Verification items for the finished model (mm, model axes). Face numbers are marked on the shaded views. A direction names the side the tool comes from. Round coordinates to 2 decimals unless told otherwise and drop trailing zeros. Write each loop counter-clockwise with the first axis right and the second up, starting at its lowest first coordinate (ties: lowest second). Pieces come first, ordered by that corner, then holes. Notation, with made-up numbers: M -18.5,49 L 21.5,49 A32 cw 21.5,77 Z; hole C 83.5,-21.75 d10. An arc over 180 degrees is marked long. One line per question, with ' | ' between items.
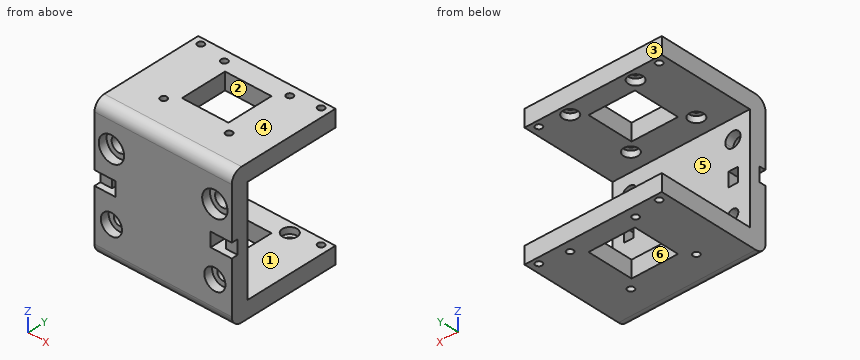
from build123d import *

# Parameters (mm, degrees)
F0_W      = 65
F0_H      = 50
F0_W_2    = 45
F0_H_2    = 6.7
F1_DEPTH  = 8
F2_R      = 6
F2_R_2    = 3.6
F2_R_3    = 5
F2_R_4    = 2.55
F3_DEPTH  = 4
F4_W      = 5.5
F4_H      = 6.7
F5_DEPTH  = 3
F6_DEPTH  = 8
F7_DEPTH  = 8
F8_W      = 65
F8_H      = 8
F9_DEPTH  = 45
F10_W     = 22
F10_H     = 22
F10_R     = 1.55
F11_DEPTH = 100
F12_R     = 3.5
F12_R_2   = 1.55
F13_DEPTH = 3
F14_R     = 3.5
F14_R_2   = 1.55
F15_DEPTH = 3
F16_R     = 5


with BuildPart() as f1:
    # F0 (on Front) → F1 (new body)
    with BuildSketch(Plane.XZ):
        Rectangle(F0_W, F0_H)
        with BuildLine():
            ThreePointArc((-24.5, 12.35), (-27.0455844123, 18.4955844123), (-20.9, 15.95))
            Line((-20.9, 15.95), (20.9, 15.95))
            ThreePointArc((20.9, 15.95), (24.5, 19.55), (28.1, 15.95))
            ThreePointArc((28.1, 15.95), (27.0455844123, 13.4044155877), (24.5, 12.35))
            Line((24.5, 12.35), (24.5, 3.35))
            Line((24.5, 3.35), (27, 3.35))
            Line((27, 3.35), (27, -3.35))
            Line((27, -3.35), (24.5, -3.35))
            Line((24.5, -3.35), (24.5, -13.4))
            ThreePointArc((24.5, -13.4), (26.303122292, -14.146877708), (27.05, -15.95))
            ThreePointArc((27.05, -15.95), (24.5, -18.5), (21.95, -15.95))
            Line((21.95, -15.95), (-21.95, -15.95))
            ThreePointArc((-21.95, -15.95), (-26.303122292, -17.753122292), (-24.5, -13.4))
            Line((-24.5, -13.4), (-24.5, -3.35))
            Line((-24.5, -3.35), (-27, -3.35))
            Line((-27, -3.35), (-27, 3.35))
            Line((-27, 3.35), (-24.5, 3.35))
            Line((-24.5, 3.35), (-24.5, 12.35))
        make_face(mode=Mode.SUBTRACT)
        with BuildLine():
            Line((20.9, 15.95), (-20.9, 15.95))
            ThreePointArc((-20.9, 15.95), (-21.9544155877, 13.4044155877), (-24.5, 12.35))
            Line((-24.5, 12.35), (-24.5, 3.35))
            Line((-24.5, 3.35), (-22.5, 3.35))
            Line((-22.5, 3.35), (22.5, 3.35))
            Line((22.5, 3.35), (24.5, 3.35))
            Line((24.5, 3.35), (24.5, 12.35))
            ThreePointArc((24.5, 12.35), (21.9544155877, 13.4044155877), (20.9, 15.95))
        make_face()
        with BuildLine():
            Line((-22.5, -3.35), (-24.5, -3.35))
            Line((-24.5, -3.35), (-24.5, -13.4))
            ThreePointArc((-24.5, -13.4), (-22.696877708, -14.146877708), (-21.95, -15.95))
            Line((-21.95, -15.95), (21.95, -15.95))
            ThreePointArc((21.95, -15.95), (22.696877708, -14.146877708), (24.5, -13.4))
            Line((24.5, -13.4), (24.5, -3.35))
            Line((24.5, -3.35), (22.5, -3.35))
            Line((22.5, -3.35), (-22.5, -3.35))
        make_face()
        Rectangle(F0_W_2, F0_H_2)
    extrude(amount=F1_DEPTH)

    # F2 (on face) → F3 (cut)
    with BuildSketch(Plane.XZ.offset(8)):
        with Locations((24.5, 15.95)):
            Circle(F2_R)
        with Locations((24.5, 15.95)):
            Circle(F2_R_2, mode=Mode.SUBTRACT)
        with Locations((-24.5, 15.95)):
            Circle(F2_R)
        with Locations((-24.5, 15.95)):
            Circle(F2_R_2, mode=Mode.SUBTRACT)
        with Locations((-24.5, -15.95)):
            Circle(F2_R_3)
        with Locations((-24.5, -15.95)):
            Circle(F2_R_4, mode=Mode.SUBTRACT)
        with Locations((24.5, -15.95)):
            Circle(F2_R_3)
        with Locations((24.5, -15.95)):
            Circle(F2_R_4, mode=Mode.SUBTRACT)
    extrude(amount=-F3_DEPTH, mode=Mode.SUBTRACT)

    # F4 (on face) → F5 (cut)
    with BuildSketch(Plane.XZ.offset(8)):
        with Locations((29.75, 0)):
            Rectangle(F4_W, F4_H)
        with Locations((-29.75, 0)):
            Rectangle(F4_W, F4_H)
    extrude(amount=-F5_DEPTH, mode=Mode.SUBTRACT)

    # F6 (add): a face of the model
    f6_faces = [f1.faces().sort_by_distance(p)[0] for p in [
        (0, -4, -25),
    ]]
    extrude(f6_faces, amount=F6_DEPTH)

    # F7 (add): a face of the model
    f7_faces = [f1.faces().sort_by_distance(p)[0] for p in [
        (0, -4, 25),
    ]]
    extrude(f7_faces, amount=F7_DEPTH)

    # F8 (on face) → F9 (join)
    with BuildSketch(Plane(origin=(0, 0, 0), x_dir=(-1, 0, 0), z_dir=(0, 1, 0))):
        with Locations((0, 29)):
            Rectangle(F8_W, F8_H)
        with Locations((0, -29)):
            Rectangle(F8_W, F8_H)
    extrude(amount=F9_DEPTH)

    # F10 (on face) → F11 (cut)
    with BuildSketch(Plane.XY.offset(33)):
        with BuildLine():
            Line((15.5, 9), (13.95, 9))
            ThreePointArc((13.95, 9), (15.5, 7.45), (17.05, 9))
            ThreePointArc((17.05, 9), (16.5960155108, 10.0960155108), (15.5, 10.55))
            Line((15.5, 10.55), (15.5, 9))
        make_face()
        with BuildLine():
            ThreePointArc((15.5, 10.55), (14.4039844892, 10.0960155108), (13.95, 9))
            Line((13.95, 9), (15.5, 9))
            Line((15.5, 9), (15.5, 10.55))
        make_face()
        with BuildLine():
            ThreePointArc((-15.5, 10.55), (-16.5960155108, 7.9039844892), (-13.95, 9))
            Line((-13.95, 9), (-15.5, 9))
            Line((-15.5, 9), (-15.5, 10.55))
        make_face()
        with BuildLine():
            Line((-15.5, 9), (-13.95, 9))
            ThreePointArc((-13.95, 9), (-14.4039844892, 10.0960155108), (-15.5, 10.55))
            Line((-15.5, 10.55), (-15.5, 9))
        make_face()
        with BuildLine():
            Line((15.5, 40), (15.5, 38.45))
            ThreePointArc((15.5, 38.45), (16.5960155108, 38.9039844892), (17.05, 40))
            ThreePointArc((17.05, 40), (15.5, 41.55), (13.95, 40))
            Line((13.95, 40), (15.5, 40))
        make_face()
        with BuildLine():
            ThreePointArc((13.95, 40), (14.4039844892, 38.9039844892), (15.5, 38.45))
            Line((15.5, 38.45), (15.5, 40))
            Line((15.5, 40), (13.95, 40))
        make_face()
        with BuildLine():
            ThreePointArc((-13.95, 40), (-16.5960155108, 41.0960155108), (-15.5, 38.45))
            Line((-15.5, 38.45), (-15.5, 40))
            Line((-15.5, 40), (-13.95, 40))
        make_face()
        with BuildLine():
            Line((-15.5, 40), (-15.5, 38.45))
            ThreePointArc((-15.5, 38.45), (-14.4039844892, 38.9039844892), (-13.95, 40))
            Line((-13.95, 40), (-15.5, 40))
        make_face()
        with Locations((0, 24.5)):
            Rectangle(F10_W, F10_H)
        with Locations((28.5, 42)):
            Circle(F10_R)
        with BuildLine():
            ThreePointArc((-26.95, 42), (-28.5, 43.55), (-30.05, 42))
            ThreePointArc((-30.05, 42), (-28.5, 40.45), (-26.95, 42))
        make_face()
    extrude(amount=-F11_DEPTH, mode=Mode.SUBTRACT)

    # F12 (on face) → F13 (cut)
    with BuildSketch(Plane(origin=(0, 0, 25), x_dir=(1, 0, 0), z_dir=(0, 0, -1))):
        with Locations((-15.5, -40)):
            Circle(F12_R)
        with Locations((-15.5, -40)):
            Circle(F12_R_2, mode=Mode.SUBTRACT)
        with Locations((-15.5, -9)):
            Circle(F12_R)
        with Locations((-15.5, -9)):
            Circle(F12_R_2, mode=Mode.SUBTRACT)
        with Locations((15.5, -9)):
            Circle(F12_R)
        with Locations((15.5, -9)):
            Circle(F12_R_2, mode=Mode.SUBTRACT)
        with Locations((15.5, -40)):
            Circle(F12_R)
        with Locations((15.5, -40)):
            Circle(F12_R_2, mode=Mode.SUBTRACT)
    extrude(amount=-F13_DEPTH, mode=Mode.SUBTRACT)

    # F14 (on face) → F15 (cut)
    with BuildSketch(Plane.XY.offset(-25)):
        with Locations((15.5, 9)):
            Circle(F14_R)
        with Locations((15.5, 9)):
            Circle(F14_R_2, mode=Mode.SUBTRACT)
        with Locations((15.5, 40)):
            Circle(F14_R)
        with Locations((15.5, 40)):
            Circle(F14_R_2, mode=Mode.SUBTRACT)
        with Locations((-15.5, 40)):
            Circle(F14_R)
        with Locations((-15.5, 40)):
            Circle(F14_R_2, mode=Mode.SUBTRACT)
        with Locations((-15.5, 9)):
            Circle(F14_R)
        with Locations((-15.5, 9)):
            Circle(F14_R_2, mode=Mode.SUBTRACT)
    extrude(amount=-F15_DEPTH, mode=Mode.SUBTRACT)

    # F16
    f16_edges = [f1.edges().sort_by_distance(p)[0] for p in [
        (0, -8, -33),
        (0, -8, 33),
    ]]
    fillet(f16_edges, radius=F16_R)


solid = f1.part
1. Thickness scan on line 1 (X direction, y = 9, z = -31.75); line 2 (Y direction, x = 15.5, z = -26.4); line 3 (Z direction, x = -24.5, y = -3.1). Record the ranges inside material, lowest first.
Results:
line 1: x = -32.5 to -17.05, -13.95 to 13.95, 17.05 to 32.5 | line 2: y = -8 to 5.5, 12.5 to 36.5, 43.5 to 45 | line 3: z = -33 to -18.5, -13.4 to -3.35, 3.35 to 12.35, 19.55 to 33
2. Mould release check, pull along Z, two halves, no side actions. Record for the marked faces 4, 5 and 6: pulls with the +Z half, pulls with the -Z half, needs draft (parallel to the pull), parting line crosses it, or undercut.
Results:
face 4: pulls with the +Z half | face 5: undercut | face 6: needs draft
3. Section check A-A, the plane y = 17.5. Record the cut outline in (x, z).
Results:
outline: M -32.5,-33 L -11,-33 L -11,-25 L -32.5,-25 Z; M -32.5,25 L -11,25 L -11,33 L -32.5,33 Z; M 11,-33 L 32.5,-33 L 32.5,-25 L 11,-25 Z; M 11,25 L 32.5,25 L 32.5,33 L 11,33 Z
4. Section check C-C, the plane z = -14.5. Record the cut outline in (x, y).
Results:
outline: M -32.5,-8 L -29.29,-8 L -29.29,-4 L -26.6,-4 L -26.6,0 L -32.5,0 Z; M -22.4,-4 L -19.71,-4 L -19.71,-8 L 19.71,-8 L 19.71,-4 L 22.4,-4 L 22.4,0 L -22.4,0 Z; M 26.6,-4 L 29.29,-4 L 29.29,-8 L 32.5,-8 L 32.5,0 L 26.6,0 Z
5. Go/stop test with flat-tipped pins: P1, Ø9.5, axis at x = 24.5, z = 18, coming from the -Y side; P2, Ø4, axis at x = 17.5, z = 0.5, coming from the +Y side; P3, Ø1.5, axis at x = 24, z = 12, coming from the -Y side. Record where each tip stops, or that it passes through.
Results:
P1: stops at y = -8 | P2: stops at y = 0 | P3: stops at y = -4
6. Section check B-B, the plane x = -1. Record the cut outline in (y, z), then the cut area to 3 significant figures.
Results:
outline: M -8,-28 A5 ccw -3,-33 L 13.5,-33 L 13.5,-25 L 0,-25 L 0,25 L 13.5,25 L 13.5,33 L -3,33 A5 ccw -8,28 Z; M 35.5,-33 L 45,-33 L 45,-25 L 35.5,-25 Z; M 35.5,25 L 45,25 L 45,33 L 35.5,33 Z | area: 885 mm2
7. Tool access check on the marked faces 1, 2 and 3. Record the directions out of +Z, -Z, +X, -X, +Y, -Y that give a thin tool (end or side, any length) a straight path to the whole face; none if there is none.
Results:
face 1: +X, -X, +Y | face 2: +Z, -Z | face 3: +Z, -Z, +X, -X, +Y
8. Section check D-D, the plane z = -5. Record the cut outline in (x, y).
Results:
outline: M -32.5,-8 L 32.5,-8 L 32.5,0 L -32.5,0 Z
